Here's how the part is built. I have some questions about the finished solid (model axes, mm). Face numbers are marked on the shaded views. A direction names the side the tool comes from. Round coordinates to 2 decimals unless told otherwise and drop trailing zeros. Loops run counter-clockwise (first coordinate to the right, second up) from the corner with the lowest first, then second, coordinate; pieces in that order, holes last. Notation, with made-up numbers: M -6,81 L 10,81 A16 ccw 10,107 Z; hole C -13.75,-32.5 d3. An arc over 180 degrees is marked long. Use a Markdown table: item, result.
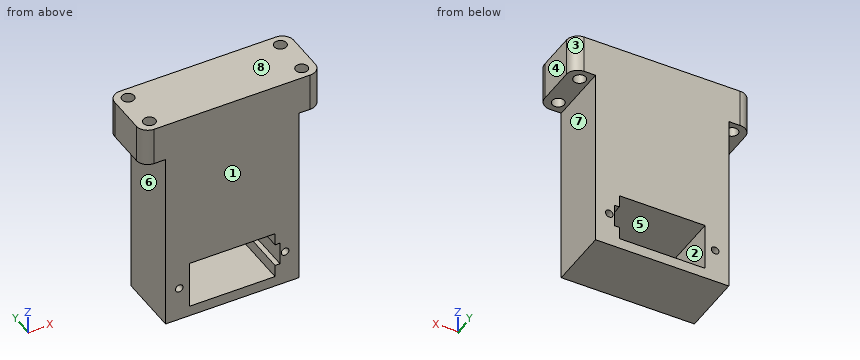
from build123d import *

# Parameters (mm, degrees)
SKETCH_2_W          = 35
SKETCH_2_H          = 18
SKETCH_2_W_2        = 22.5
SKETCH_2_H_2        = 12.5
EXTRUDE_1_DEPTH     = 16.1
SKETCH_3_R          = 1
CUT_EXTRUDE_1_DEPTH = 26.425577673
SKETCH_8_W          = 1.3
SKETCH_8_H          = 6
CUT_EXTRUDE_2_DEPTH = 26.425577673
SKETCH_9_W          = 6
SKETCH_9_H          = 16.1
SKETCH_9_R          = 1.6
EXTRUDE_4_DEPTH     = 10
EXTRUDE_4_2_DEPTH   = 10
SKETCH_10_W         = 35
SKETCH_10_H         = 16.1
EXTRUDE_5_DEPTH     = 40
FILLET_1_R          = 3


with BuildPart() as part:
    # Sketch 2 → Extrude 1 (new body)
    with BuildSketch(Plane(origin=(0, 0, 0), x_dir=(1, 0, 0), z_dir=(0, 1, 0))):
        Rectangle(SKETCH_2_W, SKETCH_2_H)
        Rectangle(SKETCH_2_W_2, SKETCH_2_H_2, mode=Mode.SUBTRACT)
    extrude(amount=EXTRUDE_1_DEPTH)

    # Sketch 3 → Cut-Extrude 1 (cut, through all)
    with BuildSketch(Plane(origin=(0, 16.1, 0), x_dir=(1, 0, 0), z_dir=(0, 1, 0))):
        with Locations(Location((-13.9, 0, 0), (0, 0, 270))):
            Circle(SKETCH_3_R)
        with Locations(Location((13.9, 0, 0), (0, 0, 270))):
            Circle(SKETCH_3_R)
    extrude(amount=-CUT_EXTRUDE_1_DEPTH, mode=Mode.SUBTRACT)

    # Sketch 8 → Cut-Extrude 2 (cut, through all)
    with BuildSketch(Plane(origin=(0, 16.1, 0), x_dir=(1, 0, 0), z_dir=(0, 1, 0))):
        with Locations((11.9, 0)):
            Rectangle(SKETCH_8_W, SKETCH_8_H)
    extrude(amount=-CUT_EXTRUDE_2_DEPTH, mode=Mode.SUBTRACT)



with BuildPart() as body_2:
    # Sketch 9 → Extrude 4 (new body)
    with BuildSketch(Plane.XY.offset(49)):
        with Locations((20.5, 8.05)):
            Rectangle(SKETCH_9_W, SKETCH_9_H)
        with Locations((20, 3.1)):
            Circle(SKETCH_9_R, mode=Mode.SUBTRACT)
        with Locations((20, 13.1)):
            Circle(SKETCH_9_R, mode=Mode.SUBTRACT)
    extrude(amount=-EXTRUDE_4_DEPTH)


with BuildPart() as body_3:
    # Sketch 9 → Extrude 4 2 (new body)
    with BuildSketch(Plane.XY.offset(49)):
        with Locations((-20.5, 8.05)):
            Rectangle(SKETCH_9_W, SKETCH_9_H)
        with Locations((-20, 3.1)):
            Circle(SKETCH_9_R, mode=Mode.SUBTRACT)
        with Locations((-20, 13.1)):
            Circle(SKETCH_9_R, mode=Mode.SUBTRACT)
    extrude(amount=-EXTRUDE_4_2_DEPTH)


with BuildPart() as part_1:
    add(part.part)

    add(body_2.part)  # Extrude 5 merges body 2

    add(body_3.part)  # Extrude 5 merges body 3
    # Sketch 10 → Extrude 5 (add)
    with BuildSketch(Plane.XY.offset(49)):
        with Locations((0, 8.05)):
            Rectangle(SKETCH_10_W, SKETCH_10_H)
    extrude(amount=-EXTRUDE_5_DEPTH)

    # Fillet 1
    fillet_1_edges = [part_1.edges().sort_by_distance(p)[0] for p in [
        (23.5, 16.1, 44),
        (23.5, 0, 44),
        (-23.5, 16.1, 44),
        (-23.5, 0, 44),
    ]]
    fillet(fillet_1_edges, radius=FILLET_1_R)


solid = part_1.part
1. I need wall thicknesses on probe 1 along Y at (x, z) = (20, 47); probe 2 along X at (y, z) = (10.75, 0); probe 3 along X at (y, z) = (13, 6). Which ranges of each line are inside material? Lowest first, please. Write a range as from..to.
Answer sheet:
| item | result |
|---|---|
| probe 1 | 0..1.5, 4.7..11.5, 14.7..16.1 |
| probe 2 | -17.5..-14.9, -12.9..-11.25, 12.55..12.9, 14.9..17.5 |
| probe 3 | -17.5..-11.25, 11.25..17.5 |
2. Imagine slicing it at A-A, the plane y = 14. Write out the boundary of the cut face in (x, z).
Answer sheet:
| item | result |
|---|---|
| outline | M -23.36,39 L -21.32,39 L -21.32,49 L -23.36,49 Z; M -18.68,39 L -17.5,39 L -17.5,-9 L 17.5,-9 L 17.5,39 L 18.68,39 L 18.68,49 L -18.68,49 Z; M 21.32,39 L 23.36,39 L 23.36,49 L 21.32,49 Z; hole C -13.9,0 d2; hole M -11.25,-6.25 L 11.25,-6.25 L 11.25,-3 L 12.55,-3 L 12.55,3 L 11.25,3 L 11.25,6.25 L -11.25,6.25 Z; hole C 13.9,0 d2 |
3. Imagine slicing it at D-D, the plane y = 9.75. Write out the boundary of the cut face in (x, z).
Answer sheet:
| item | result |
|---|---|
| outline | M -23.5,39 L -17.5,39 L -17.5,-9 L 17.5,-9 L 17.5,39 L 23.5,39 L 23.5,49 L -23.5,49 Z; hole C -13.9,0 d2; hole M -11.25,-6.25 L 11.25,-6.25 L 11.25,-3 L 12.55,-3 L 12.55,3 L 11.25,3 L 11.25,6.25 L -11.25,6.25 Z; hole C 13.9,0 d2 |
4. We'd pull the mould along X, two halves only. Please class the marked faces 1, 2 and 3: +X half, -X half, draft (parallel to the pull), parting line (faces both ways), or undercut.
Answer sheet:
| item | result |
|---|---|
| face 1 | draft |
| face 2 | undercut |
| face 3 | +X half |
5. Imagine slicing it at B-B, the plane z = 0. Write out the boundary of the cut face in (x, y).
Answer sheet:
| item | result |
|---|---|
| outline | M -17.5,0 L -14.9,0 L -14.9,16.1 L -17.5,16.1 Z; M -12.9,0 L -11.25,0 L -11.25,16.1 L -12.9,16.1 Z; M 12.55,0 L 12.9,0 L 12.9,16.1 L 12.55,16.1 Z; M 14.9,0 L 17.5,0 L 17.5,16.1 L 14.9,16.1 Z |
6. Which directions (+Z, -Z, +X, -X, +Y, -Y) give clear straight access to the entire face, cutting with the end or side of a thin tool? Please do the marked faces 4, 5, 6, 7 and 8.
Answer sheet:
| item | result |
|---|---|
| face 4 | +Z, -Z, +X, +Y, -Y |
| face 5 | +Y, -Y |
| face 6 | -Z, -X, +Y, -Y |
| face 7 | -Z, +X, +Y, -Y |
| face 8 | +Z, +X, -X, +Y, -Y |
7. Imagine slicing it at C-C, the plane x = -13.9. Write out the boundary of the cut face in (y, z), then the cut area to 3 significant figures.
Answer sheet:
| item | result |
|---|---|
| outline | M 0,-9 L 16.1,-9 L 16.1,-1 L 0,-1 Z; M 0,1 L 16.1,1 L 16.1,49 L 0,49 Z |
| area | 902 mm2 |
8. For pin 1 Ø4 at (x, y) = (20, 3.1) entering from -Z; pin 2 Ø5 at (x, y) = (-19.5, 10) entering from -Z; pin 3 Ø1 at (y, z) = (11, -4.5) entering from -X; pin 4 Ø4 at (y, z) = (4.5, -2.5) entering from +X, each with a flat end and sliding along its axis, tell me the tip position at first contact or that it passes through.
Answer sheet:
| item | result |
|---|---|
| pin 1 | z = 39 |
| pin 2 | z = -9 |
| pin 3 | x = -17.5 |
| pin 4 | x = 17.5 |
